The listing builds one solid part. Answer for the finished solid, in the listing's coordinates (mm). Face numbers are marked on the shaded views. A direction names the side the tool comes from. Round coordinates to 2 decimals unless told otherwise and drop trailing zeros. Write each loop counter-clockwise with the first axis right and the second up, starting at its lowest first coordinate (ties: lowest second). Pieces come first, ordered by that corner, then holes.
Item 1: Find section C-C on y = 33. Give the vertices of the cut face in (x, z) (3 decimals), then the cut area to 3 significant figures.
Item 2: Each of these flat-tipped pins is pushed along its axis until it touches: pin 1 (11 mm diameter, centred on y = 107.5, z = 139.5, fed in from +X); pin 2 (12 mm diameter, centred on x = 123.5, y = 114.5, fed in from +Z). Where does it stop, or does it pass through?
Item 3: Find section D-D on y = 106. Give the vertices of the cut face in (x, z) (3 decimals), then the cut area to 3 significant figures.
Item 4: Find section A-A on x = 37.5. Give the vertices of the cut face in (y, z).
Item 5: A tool of negligible diameter and unlimited length cuts with its end or side. For the marked faces 4, 5 and 6, from which of +Z, -Z, +X, -X, +Y, -Y can it reach the whole face along a straight path? Write none if from no direction.
Item 6: For a pull along Z with two mould halves and no side action, classify the marked faces 1, 2 and 3 as +Z half, -Z half, draft (parallel to the pull), parting line (faces both ways), or undercut.
Item 7: Find the intervals of material crossed by probe 1 along Y at (x, z) = (34, 69.5); probe 2 along Y at (x, z) = (62, 99.5); probe 3 along Y at (x, z) = (67.5, 135), in increasing order.
```python
from build123d import *

# Parameters (mm, degrees)
SKETCH1_W           = 150
SKETCH1_H           = 150
SKETCH1_W_2         = 65
SKETCH1_H_2         = 95
BOSS_EXTRUDE2_DEPTH = 152
CHAMFER1_SIZE       = 78.48885271
SKETCH4_W           = 148.25
SKETCH4_H           = 111
CUT_EXTRUDE5_DEPTH  = 19
SKETCH5_W           = 136.25
SKETCH5_H           = 84
CUT_EXTRUDE6_DEPTH  = 81
SKETCH6_W           = 10
SKETCH6_H           = 10
CUT_EXTRUDE7_DEPTH  = 40
SKETCH7_W           = 10
SKETCH7_H           = 10
CUT_EXTRUDE8_DEPTH  = 40
SKETCH10_W          = 40
SKETCH10_H          = 6
CUT_EXTRUDE10_DEPTH = 10


with BuildPart() as part:
    # Sketch1 → Boss-Extrude2 (new body)
    with BuildSketch(Plane.XY):
        with Locations((75, 75)):
            Rectangle(SKETCH1_W, SKETCH1_H)
        with Locations((37.5, 52.5)):
            Rectangle(SKETCH1_W_2, SKETCH1_H_2, mode=Mode.SUBTRACT)
    extrude(amount=BOSS_EXTRUDE2_DEPTH)

    # Chamfer1
    chamfer1_edges = [part.edges().sort_by_distance(p)[0] for p in [
        (150, 150, 76),
    ]]
    chamfer(chamfer1_edges, length=CHAMFER1_SIZE)

    # Sketch4 → Cut-Extrude5 (cut)
    with BuildSketch(Plane(origin=(110.755573645, 110.755573645, 0), x_dir=(0, 0, -1), z_dir=(0.7071067811865489, 0.7071067811865461, 0))):
        with Locations((-76, 0.001948307)):
            Rectangle(SKETCH4_W, SKETCH4_H)
    extrude(amount=-CUT_EXTRUDE5_DEPTH, mode=Mode.SUBTRACT)

    # Sketch5 → Cut-Extrude6 (cut)
    with BuildSketch(Plane(origin=(97.320544802, 97.320544802, 0), x_dir=(0, 0, -1), z_dir=(0.707106781186549, 0.707106781186546, 0))):
        with Locations((-76, 0.001948307)):
            Rectangle(SKETCH5_W, SKETCH5_H)
    extrude(amount=-CUT_EXTRUDE6_DEPTH, mode=Mode.SUBTRACT)

    # Sketch6 → Cut-Extrude7 (cut)
    with BuildSketch(Plane.XY.offset(152)):
        with Locations((15, 105)):
            Rectangle(SKETCH6_W, SKETCH6_H)
    extrude(amount=-CUT_EXTRUDE7_DEPTH, mode=Mode.SUBTRACT)

    # Sketch7 → Cut-Extrude8 (cut)
    with BuildSketch(Plane.XY.offset(152)):
        with Locations((60, 105)):
            Rectangle(SKETCH7_W, SKETCH7_H)
    extrude(amount=-CUT_EXTRUDE8_DEPTH, mode=Mode.SUBTRACT)

    # Sketch10 → Cut-Extrude10 (cut)
    with BuildSketch(Plane.XZ.offset(-100)):
        with Locations((40, 115)):
            Rectangle(SKETCH10_W, SKETCH10_H)
    extrude(amount=-CUT_EXTRUDE10_DEPTH, mode=Mode.SUBTRACT)


solid = part.part
```
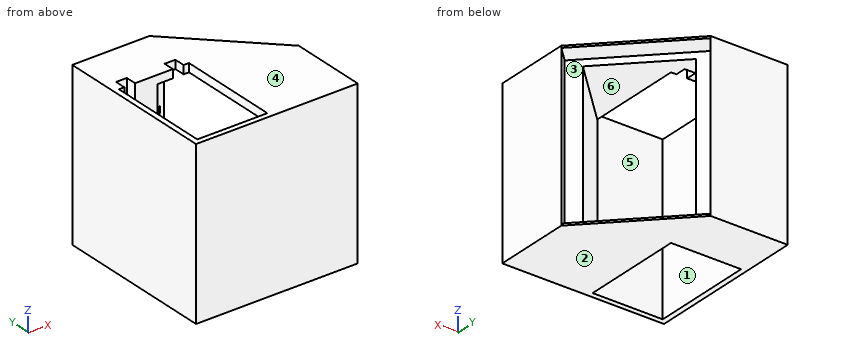
Check values:
1. outline: (0, 0) - (5, 0) - (5, 152) - (0, 152) - close; (70, 0) - (150, 0) - (150, 152) - (70, 152) - (70, 144.125) - (92.394, 144.125) - (92.394, 7.875) - (70, 7.875) - close
1. area: 9,870 mm2
2. pin 1: stops at x = 90.12
2. pin 2: passes through
3. outline: (0, 0) - (115.511, 0) - (115.511, 1.875) - (88.641, 1.875) - (88.641, 7.875) - (46.6, 7.875) - (46.6, 112) - (10, 112) - (10, 152) - (0, 152) - close; (20, 118) - (46.6, 118) - (46.6, 144.125) - (55, 144.125) - (55, 152) - (20, 152) - close; (65, 144.125) - (88.641, 144.125) - (88.641, 150.125) - (115.511, 150.125) - (115.511, 152) - (65, 152) - close
3. area: 7,210 mm2
4. outline: (0, 0) - (5, 0) - (5, 152) - (0, 152) - close; (100, 0) - (150, 0) - (150, 152) - (100, 152) - (100, 118) - (110, 118) - (110, 112) - (100, 112) - close
5. face 4: +Z, +X, -X, +Y, -Y
5. face 5: +Z, -Z
5. face 6: none
6. face 1: draft
6. face 2: -Z half
6. face 3: undercut
7. probe 1: y = 0 to 5, 100 to 150
7. probe 2: y = 0 to 5, 121.4 to 132.64, 140.49 to 150
7. probe 3: y = 0 to 5, 126.9 to 127.14, 145.99 to 150
